Part model, mm, in its own coordinate system. A direction names the side the tool comes from. Round coordinates to 2 decimals unless told otherwise and drop trailing zeros. Loops run counter-clockwise (first coordinate to the right, second up) from the corner with the lowest first, then second, coordinate; pieces in that order, holes last. Notation, with made-up numbers: M -34.75,-33.75 L -15.75,-33.75 A29 cw -15.75,-8.75 Z; hole C 52,22.25 d5. An arc over 180 degrees is marked long. Put each result on its own line as item: value. Start each with the question number.
1) Probe line 1 along X through (y, z) = (0.7, 0); line 2 along Y through (x, z) = (1, 1.5); line 3 along Y through (x, z) = (-14, 1.75). List the from-to ranges inside material, lowest first.
2) Which spindle directions (+Z, -Z, +X, -X, +Y, -Y) get a long thin tool onto all of the face, cutting with end or side? Do faces 1 (the cylindrical face through (-1.256, 3.623, -1.638)), 2 (the cylindrical face through (-2.44, 1.25, -0.54)), 3 (the cylindrical face through (8.416, 3.392, -0.065)). Say none if no direction does.
3) Slice it at A-A on x = 0. Give the cut face in (y, z).
4) Drop flat-ended pins along their axis: pin 1 Ø3 at (x, z) = (0, 0) entering from +Y; pin 2 Ø4 at (x, z) = (-5.5, 0.5) entering from -Y; pin 3 Ø1.4 at (x, z) = (0, 0) entering from -Y; pin 4 Ø2 at (y, z) = (3, 1.5) entering from -X. Give the stop position or say it passes through.
5) Slice it at C-C on z = 0. State how many separate pieces and enclosed holes the cut face has, then the cut area to 3 significant figures.
6) Pull direction Z, two halves, no side cores. Call faces 4 (the flat face through (8.15, 3.39, -3.01)), 5 (the flat face through (-1, 2.997, 1)), 6 (the flat face through (-8.15, 3.39, 3.01)): +Z half, -Z half, draft (parallel to the pull), parting line (faces both ways), or undercut.
7) Slice it at D-D on z = -1.75. Give the cut face in (x, y), then the cut area to 3 significant figures.
8) Slice it at B-B on y = 0.7. Give the cut face in (x, z).
```python
from build123d import *

# Parameters (mm, degrees)
SKETCH1_R           = 3.3655
SKETCH1_R_2         = 2.5
BOSS_EXTRUDE1_DEPTH = 2.54
SKETCH2_R           = 0.5
SKETCH2_R_2         = 1.143
BOSS_EXTRUDE2_DEPTH = 1.7272
FILLET1_R           = 12.7
CUT_EXTRUDE1_START  = -1.27
SKETCH3_R           = 2.06375
SKETCH3_R_2         = 1.143
CUT_EXTRUDE1_DEPTH  = 1.27


with BuildPart() as part:
    # Sketch1 → Boss-Extrude1 (new body)
    with BuildSketch(Plane(origin=(0, 0, 0), x_dir=(1, 0, 0), z_dir=(0, 1, 0))):
        with Locations(Location((0, 0, 0), (0, 0, 270))):
            Circle(SKETCH1_R)
        with Locations(Location((0, 0, 0), (0, 0, 270))):
            Circle(SKETCH1_R_2, mode=Mode.SUBTRACT)
    extrude(amount=BOSS_EXTRUDE1_DEPTH)

    # Sketch2 → Boss-Extrude2 (add)
    with BuildSketch(Plane(origin=(0, 2.54, 0), x_dir=(1, 0, 0), z_dir=(0, 1, 0))):
        with BuildLine():
            Line((0, 3.8227), (15.229633673, 2.30634634))
            ThreePointArc((15.229633673, 2.30634634), (17.31775, 0), (15.229633673, -2.30634634))
            Line((15.229633673, -2.30634634), (0, -3.8227))
            Line((0, -3.8227), (-15.229633673, -2.30634634))
            ThreePointArc((-15.229633673, -2.30634634), (-17.31775, 0), (-15.229633673, 2.30634634))
            Line((-15.229633673, 2.30634634), (0, 3.8227))
        make_face()
        with Locations(Location((-10.46, 0, 0), (0, 0, 270))):
            Circle(SKETCH2_R, mode=Mode.SUBTRACT)
        with Locations(Location((-7.92, 0, 0), (0, 0, 270))):
            Circle(SKETCH2_R, mode=Mode.SUBTRACT)
        with Locations(Location((-5.38, 0, 0), (0, 0, 270))):
            Circle(SKETCH2_R, mode=Mode.SUBTRACT)
        with Locations(Location((15, 0, 0), (0, 0, 270))):
            Circle(SKETCH2_R, mode=Mode.SUBTRACT)
        with Locations(Location((5.38, 0, 0), (0, 0, 270))):
            Circle(SKETCH2_R, mode=Mode.SUBTRACT)
        with Locations(Location((7.92, 0, 0), (0, 0, 270))):
            Circle(SKETCH2_R, mode=Mode.SUBTRACT)
        with Locations(Location((-13, 0, 0), (0, 0, 270))):
            Circle(SKETCH2_R, mode=Mode.SUBTRACT)
        with Locations(Location((-15, 0, 0), (0, 0, 270))):
            Circle(SKETCH2_R, mode=Mode.SUBTRACT)
        with Locations(Location((0, 0, 0), (0, 0, 270))):
            Circle(SKETCH2_R_2, mode=Mode.SUBTRACT)
        with Locations(Location((10.46, 0, 0), (0, 0, 270))):
            Circle(SKETCH2_R, mode=Mode.SUBTRACT)
        with Locations(Location((13, 0, 0), (0, 0, 270))):
            Circle(SKETCH2_R, mode=Mode.SUBTRACT)
    extrude(amount=BOSS_EXTRUDE2_DEPTH)

    # Fillet1
    fillet1_edges = [part.edges().sort_by_distance(p)[0] for p in [
        (0, 3.4036, 3.8227),
        (0, 3.4036, -3.8227),
    ]]
    fillet(fillet1_edges, radius=FILLET1_R)

    # Sketch3 → Cut-Extrude1 (cut)
    with BuildSketch(Plane(origin=(0, 4.2672, 0), x_dir=(1, 0, 0), z_dir=(0, 1, 0)).offset(CUT_EXTRUDE1_START)):
        with Locations(Location((0, 0, 0), (0, 0, 270))):
            Circle(SKETCH3_R)
        with Locations(Location((0, 0, 0), (0, 0, 270))):
            Circle(SKETCH3_R_2, mode=Mode.SUBTRACT)
    extrude(amount=CUT_EXTRUDE1_DEPTH, mode=Mode.SUBTRACT)


solid = part.part
```
Recorded:
1. line 1: x = -3.37 to -2.5, 2.5 to 3.37
1. line 2: y = 2.54 to 3
1. line 3: y = 2.54 to 4.27
2. face 1: +Y
2. face 2: -Y
2. face 3: +Y, -Y
3. outline: M 0,-3.37 L 2.54,-3.37 L 2.54,-3.76 L 4.27,-3.76 L 4.27,-2.06 L 3,-2.06 L 3,-1.14 L 2.54,-1.14 L 2.54,-2.5 L 0,-2.5 Z; M 0,2.5 L 2.54,2.5 L 2.54,1.14 L 3,1.14 L 3,2.06 L 4.27,2.06 L 4.27,3.76 L 2.54,3.76 L 2.54,3.37 L 0,3.37 Z
4. pin 1: stops at y = 3
4. pin 2: stops at y = 2.54
4. pin 3: passes through
4. pin 4: stops at x = -17.26
5. separate pieces: 12
5. enclosed holes: 0
5. area: 40.7 mm2
6. face 4: -Z half
6. face 5: undercut
6. face 6: +Z half
7. outline: M -16.52,2.54 L -2.87,2.54 L -2.87,0 L -1.79,0 L -1.79,2.54 L 1.79,2.54 L 1.79,0 L 2.87,0 L 2.87,2.54 L 16.52,2.54 L 16.52,4.27 L 1.09,4.27 L 1.09,3 L -1.09,3 L -1.09,4.27 L -16.52,4.27 Z
7. area: 59.8 mm2
8. outline: C 0,0 d6.73; hole C 0,0 d5
